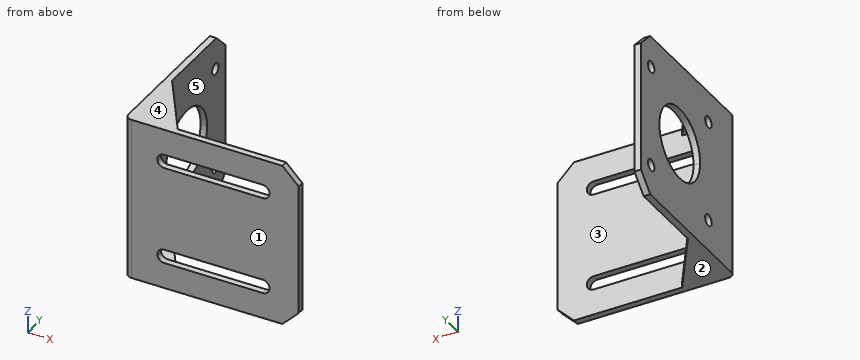
```python
from build123d import *

# Parameters (mm, degrees)
EXTRUDE_1_DEPTH = 2
SKETCH_2_R      = 1.75
EXTRUDE_2_DEPTH = 2
FILLET_1_R      = 2
EXTRUDE_3_DEPTH = 2


with BuildPart() as part:
    # 草图1 → 凸台-拉伸1 (new body)
    with BuildSketch(Plane(origin=(0, 0, 0), x_dir=(1, 0, 0), z_dir=(0, 1, 0))):
        Polygon((0, 0), (0, 25), (48, 25), (53, 20), (53, 0), align=None)
        with BuildLine():
            Line((12, 17.1), (42, 17.1))
            ThreePointArc((42, 17.1), (44.1, 15), (42, 12.9))
            Line((42, 12.9), (12, 12.9))
            ThreePointArc((12, 12.9), (9.9, 15), (12, 17.1))
        make_face(mode=Mode.SUBTRACT)
    extrude_1 = extrude(amount=EXTRUDE_1_DEPTH)

    # 草图2 → 凸台-拉伸2 (add)
    with BuildSketch(Plane.ZY):
        with BuildLine():
            Line((-25, 46), (-25, 2))
            Line((-25, 2), (0, 2))
            Line((0, 2), (0, 19))
            ThreePointArc((0, 19), (-11, 30), (0, 41))
            Line((0, 41), (0, 51))
            Line((0, 51), (-20, 51))
            Line((-20, 51), (-25, 46))
        make_face()
        with Locations((-15.5, 14.5)):
            Circle(SKETCH_2_R, mode=Mode.SUBTRACT)
        with Locations((-15.5, 45.5)):
            Circle(SKETCH_2_R, mode=Mode.SUBTRACT)
    extrude_2 = extrude(amount=-EXTRUDE_2_DEPTH)

    # 镜向2: 凸台-拉伸1, 凸台-拉伸2 across plane
    add(extrude_1.mirror(Plane.XY))
    add(extrude_2.mirror(Plane.XY))

    # 圆角1
    fillet_1_edges = [part.edges().sort_by_distance(p)[0] for p in [
        (0, 0, 0),
    ]]
    fillet(fillet_1_edges, radius=FILLET_1_R)

    # 草图4 → 凸台-拉伸3 (add)
    with BuildSketch(Plane.XY.offset(25)):
        Polygon((2, 2), (2, 22), (15, 2), align=None)
    extrude_3 = extrude(amount=-EXTRUDE_3_DEPTH)

    # 镜向4: 凸台-拉伸3 across plane
    add(extrude_3.mirror(Plane.XY))


solid = part.part
```
Here's how the part is built. I have some questions about the finished solid (model axes, mm). Face numbers are marked on the shaded views. A direction names the side the tool comes from. Coordinates: 2 decimals unless noted, no trailing zeros. Order: outer loops, then holes, each group sorted by start corner. A loop starts at its lowest first (then second) coordinate and runs counter-clockwise, first axis right, second up.
1) Imagine slicing it at D-D on z = -8.5. List the corners of the cut face in (x, y) for me.
2) Which directions (+Z, -Z, +X, -X, +Y, -Y) give clear straight access to the entire face, cutting with the end or side of a thin tool? Please do the marked faces 4 and 5.
3) We'd pull the mould along Z, two halves only. Please class the marked faces 1, 2 and 3: +Z half, -Z half, draft (parallel to the pull), parting line (faces both ways), or undercut.
4) Will these pins go through, and if not, where does the flat tip stop? pin 1 (1 mm diameter, centred on y = 8, z = -12.5, fed in from +X); pin 2 (12 mm diameter, centred on x = 11, z = 3.5, fed in from +Y).
5) I need wall thicknesses on line 1 (Y direction, x = 0.55, z = 15.5); line 2 (Y direction, x = 1.4, z = 15.5); line 3 (Z direction, x = 1, y = 45). Which ranges of each line are inside material? Lowest first, please.
6) Imagine slicing it at A-A on x = 38.5. List the corners of the cut face in (y, z) for me.
7) Imagine slicing it at B-B on y = 30. List the corners of the cut face in (x, z) for me.
8) Imagine slicing it at C-C on z = 15. List the corners of the cut face in (x, y) for me, and give its area (3 significant figures).
Response values:
1. outline: (0, 2) arc R2 ccw to (2, 0) - (53, 0) - (53, 2) - (2, 2) - (2, 23.02) - (0, 23.02) - close; (0, 36.98) - (2, 36.98) - (2, 51) - (0, 51) - close
2. face 4: +Z, +X, -X, +Y, -Y
2. face 5: +X, +Y
3. face 1: draft
3. face 2: -Z half
3. face 3: undercut
4. pin 1: stops at x = 2
4. pin 2: stops at y = 2
5. line 1: y = 0.62 to 12.75, 16.25 to 43.75, 47.25 to 51
5. line 2: y = 0.09 to 12.75, 16.25 to 43.75, 47.25 to 51
5. line 3: z = -25 to -17.18, -13.82 to 13.82, 17.18 to 25
6. outline: (0, -25) - (2, -25) - (2, -17.1) - (0, -17.1) - close; (0, -12.9) - (2, -12.9) - (2, 12.9) - (0, 12.9) - close; (0, 17.1) - (2, 17.1) - (2, 25) - (0, 25) - close
7. outline: (0, -25) - (2, -25) - (2, -11) - (0, -11) - close; (0, 11) - (2, 11) - (2, 25) - (0, 25) - close
8. outline: (0, 2) arc R2 ccw to (2, 0) - (9.9, 0) - (9.9, 2) - (2, 2) - (2, 12.82) - (0, 12.82) - close; (0, 16.18) - (2, 16.18) - (2, 43.82) - (0, 43.82) - close; (0, 47.18) - (2, 47.18) - (2, 51) - (0, 51) - close; (44.1, 0) - (53, 0) - (53, 2) - (44.1, 2) - close
8. area: 121 mm2
